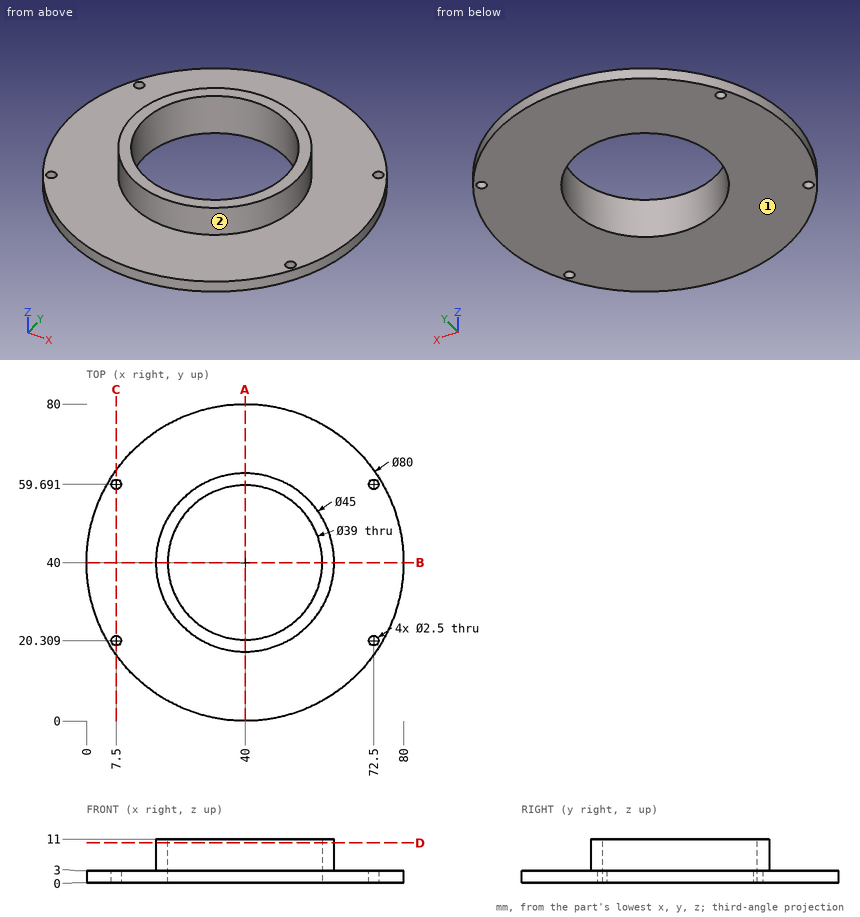
Geometry: see drawing. Coordinates: mm, zero at the bounding-box minimum. A direction names the side the tool comes from. Give positions to 0.01 mm unless a question says otherwise; leave off trailing zeros. Loops run counter-clockwise (first coordinate to the right, second up) from the corner with the lowest first, then second, coordinate; pieces in that order, holes last. Notation, with made-up numbers: (41, 30.5) - (90, 30.5) arc R25 cw to (90, 52.5) - close; hole circle Ø6 at (-36, 52). An arc over 180 degrees is marked (long way). Answer as CSV lines item,"result". Start each with the question number.
1. Ray query, L1, parallel to Y at x = 72.5, z = 0.65; L2, parallel to Z at x = 76.5, y = 24.5; L3, parallel to X at y = 51, z = 4. Return the intervals inside material, ascending.
2. Section A-A, the plane x = 40. Return loops of the section in (y, z), plus the area to 3 significant figures.
3. Pin query (flat end, axial travel): P1, Ø24, axis at x = 51, y = 38, coming from the +Z side; P2, Ø5, axis at y = 28, z = 8, coming from the -X side; P3, Ø4, axis at x = 8, y = 54, coming from the +Z side. Return the tip coordinate at first contact, or that it passes through.
4. Reachability of the marked faces 1 and 2 from +Z, -Z, +X, -X, +Y, -Y: full face, straight path, thin tool, end or side. Return the list, or none.
5. Section D-D, the plane z = 10. Return loops of the section in (x, y), plus the area to 3 significant figures.
6. Section C-C, the plane x = 7.5. Return loops of the section in (y, z).
Answers:
1,L1,"y = 16.68 to 19.06, 21.56 to 58.44, 60.94 to 63.32"
1,L2,"z = 0 to 3"
1,L3,"x = 20.37 to 23.9, 56.1 to 59.63"
2,outline,"(0, 0) - (20.5, 0) - (20.5, 11) - (17.5, 11) - (17.5, 3) - (0, 3) - close; (59.5, 0) - (80, 0) - (80, 3) - (62.5, 3) - (62.5, 11) - (59.5, 11) - close"
2,area,"171 mm2"
3,P1,"stops at z = 11"
3,P2,"stops at x = 19.6"
3,P3,"stops at z = 3"
4,face 1,"-Z, +X, -X, +Y, -Y"
4,face 2,"+Z"
5,outline,"circle Ø45 at (40, 40); hole circle Ø39 at (40, 40)"
5,area,"396 mm2"
6,outline,"(16.68, 0) - (19.06, 0) - (19.06, 3) - (16.68, 3) - close; (21.56, 0) - (58.44, 0) - (58.44, 3) - (21.56, 3) - close; (60.94, 0) - (63.32, 0) - (63.32, 3) - (60.94, 3) - close"
